Autodesk Inventor part; units mm, degrees
ref_plane "YZ Plane" through (0, 0, 0) normal (1, 0, 0) x (0, 1, 0)
ref_plane "XZ Plane" through (0, 0, 0) normal (0, 1, 0) x (-1, 0, 0)
ref_plane "XY Plane" through (0, 0, 0) normal (0, 0, 1) x (1, 0, 0)
sketch "Sketch1" plane through (0, 0, 0) normal (0, 1, 0) x (-1, 0, 0)
  line L0 (-2.6035, 25.4) -> (-6.2865, 25.4)
  line L1 (-6.2865, 25.4) -> (-6.2865, -25.4)
  line L2 (-6.2865, -25.4) -> (-2.6035, -25.4)
  line L3 (6.2865, -16.51) -> (6.2865, 16.51)
  line L4 (6.2865, 25.4) -> (-6.2865, -25.4) construction
  line L5 (-6.2865, 25.4) -> (6.2865, -25.4) construction
  arc A0 (6.2865, 16.51) -> (-2.6035, 25.4) centre (-2.6035, 16.51) ccw
  arc A1 (-2.6035, -25.4) -> (6.2865, -16.51) centre (-2.6035, -16.51) ccw
  point P0 (0, 0)
  dimension "d0" = 12.573
  dimension "d1" = 50.8
  dimension "d2" = 8.89
extrude "Extrusion1" add sketch "Sketch1" along normal blind 4.826
sketch "Sketch2" plane through (6.2865, 0, 25.4) normal (1, 0, 0) x (0, 0, -1)
  line L0 (20.3835, 2.1639) -> (30.4165, 2.1639)
  line L1 (25.4, 0) -> (20.3835, 2.1639) construction
  line L2 (25.4, 0) -> (30.4165, 2.1639) construction
  line L3 (50.8, 0) -> (0, 0)
  line L4 (20.066, 2.1639) -> (20.066, 2.3009)
  line L5 (20.066, 2.3009) -> (30.734, 2.3009)
  line L6 (30.734, 2.3009) -> (30.734, 2.1639)
  line L7 (25.4, 0) -> (20.066, 2.3009) construction
  line L8 (25.4, 0) -> (30.734, 2.3009) construction
  line L9 (30.734, -2.3009) -> (30.4165, -2.3009)
  line L10 (20.3835, -2.3009) -> (20.066, -2.3009)
  line L11 (20.066, 2.3009) -> (19.05, 2.3009)
  line L12 (19.05, 2.3009) -> (19.05, 0)
  line L13 (30.734, 2.3009) -> (31.75, 2.3009)
  line L14 (31.75, 2.3009) -> (31.75, 0)
  point P0 (20.3835, 0)
  point P1 (30.4165, 0)
  point P2 (20.066, 0)
  point P3 (30.734, 0)
extrude "Extrusion2" cut sketch "Sketch2" against normal blind 12.7
properties part number "pig_wings"
Design review of the part built by this model. Coordinates are the model's own, in mm. A direction names the side the tool comes from. Give positions to 0.01 mm unless a question says otherwise; leave off trailing zeros. Write each loop counter-clockwise with the first axis right and the second up, starting at its lowest first coordinate (ties: lowest second). Pieces come first, ordered by that corner, then holes. Notation, with made-up numbers: (68, 65.5) -> (103, 65.5) arc R14 cw to (103, 84.5) -> close; hole circle Ø10 at (49, 30). An arc over 180 degrees is marked (long way). Answer in a Markdown table with one row per item.
(1) Clearance check with flat-ended pins moving along their axes: pin 1 (2.5 mm diameter, centred on x = -2.5, y = 1.5, fed in from -Z); pin 2 (4 mm diameter, centred on x = -1.5, z = 1.5, fed in from -Y); pin 3 (2.5 mm diameter, centred on x = -1, y = 1.5, fed in from +Z). State where each tip first meets the part, or that it passes through.
Results:
| item | result |
|---|---|
| pin 1 | z = -24.52 |
| pin 2 | y = 2.3 |
| pin 3 | z = 25.08 |
(2) Consider section A-A (y = 0.6). State the section outline as (x, z) points.
Results:
| item | result |
|---|---|
| outline | (-6.29, -16.51) arc R8.89 ccw to (2.6, -25.4) -> (6.29, -25.4) -> (6.29, -6.35) -> (-6.29, -6.35) -> close; (-6.29, 6.35) -> (6.29, 6.35) -> (6.29, 25.4) -> (2.6, 25.4) arc R8.89 ccw to (-6.29, 16.51) -> close |
(3) For faces 1 (the flat face through (4, 2, 25.4)), 2 (the flat face through (0, 1, 6.35)), list the 3-axis set-ups (+Z, -Z, +X, -X, +Y, -Y) from which the entire face can be reached by the end or side of a thin tool; tool diameter is ignored.
Results:
| item | result |
|---|---|
| face 1 | +Z, +X, -X, +Y, -Y |
| face 2 | +X, -X, -Y |
(4) To check wall thickness, follow probe 1 along Y at (x, z) = (-2.75, 1); probe 2 along Z at (x, y) = (3, 1.75); probe 3 along Z at (x, y) = (2.5, 3.9). State the ranges of each line that lie inside material, in increasing order.
Results:
| item | result |
|---|---|
| probe 1 | 2.3 to 4.83 |
| probe 2 | -25.4 to -6.35, 6.35 to 25.4 |
| probe 3 | -25.4 to 25.4 |
(5) Consider section D-D (z = 3). State the section outline as (x, y) points.
Results:
| item | result |
|---|---|
| outline | (-6.29, 2.3) -> (6.29, 2.3) -> (6.29, 4.83) -> (-6.29, 4.83) -> close |
(6) Consider section C-C (y = 4.1). State the section outline as (x, z) points, then the cut area to 3 significant figures.
Results:
| item | result |
|---|---|
| outline | (-6.29, -16.51) arc R8.89 ccw to (2.6, -25.4) -> (6.29, -25.4) -> (6.29, 25.4) -> (2.6, 25.4) arc R8.89 ccw to (-6.29, 16.51) -> close |
| area | 605 mm2 |
(7) Consider section B-B (x = 4). State the section outline as (y, z) points, then the cut area to 3 significant figures.
Results:
| item | result |
|---|---|
| outline | (0, -25.4) -> (4.83, -25.4) -> (4.83, 25.4) -> (0, 25.4) -> (0, 6.35) -> (2.3, 6.35) -> (2.3, -6.35) -> (0, -6.35) -> close |
| area | 216 mm2 |
